Check sheet for the drawn part. Datum: minimum x, y, z corner. Units: mm. A direction names the side the tool comes from. Give positions to 0.01 mm unless a question says otherwise; leave off trailing zeros. Order: outer loops, then holes, each group sorted by start corner. A loop starts at its lowest first (then second) coordinate and runs counter-clockwise, first axis right, second up. Notation, with made-up numbers: M -0.5,-30.75 L 27.5,-30.75 A9 cw 27.5,-20.75 Z; hole C 12.25,72.5 d7. An arc over 180 degrees is marked long. Answer as CSV lines item,"result". Start each with the question number.
Q1. Section check A-A, the plane z = 24. Record the boundary of the cut face in (x, y), then the cut area to 3 significant figures.
Q2. Section check C-C, the plane x = 29. Record the boundary of the cut face in (y, z), then the cut area to 3 significant figures.
Q3. Thickness scan on line 1 (Z direction, x = 5, y = 8.25); line 2 (Y direction, x = 17, z = 19.5); line 3 (X direction, y = 17.5, z = 10.25). Record the ranges inside material, lowest first.
Q4. Set-up check for the marked faces 1, 2 and 3: record each of +Z, -Z, +X, -X, +Y, -Y from which the full face is reachable in a straight line by a thin tool's end or side.
Q5. Section check B-B, the plane x = 17. Record the boundary of the cut face in (y, z).
Q6. Go/stop test with flat-tipped pins: pin 1 (3.5 mm diameter, centred on y = 14.5, z = 20, fed in from -X); pin 2 (5.5 mm diameter, centred on x = 30.5, z = 21, fed in from +Y); pin 3 (5 mm diameter, centred on x = 8.5, z = 15.5, fed in from +Y). Record where each tip stops, or that it passes through.
Q7. Mould release check, pull along X, two halves, no side actions. Record for the marked faces 4, 5 and 6: +X half, -X half, draft (parallel to the pull), parting line (faces both ways), or undercut.
Q8. Section check D-D, the plane y = 13.25. Record the boundary of the cut face in (x, z), then the cut area to 3 significant figures.
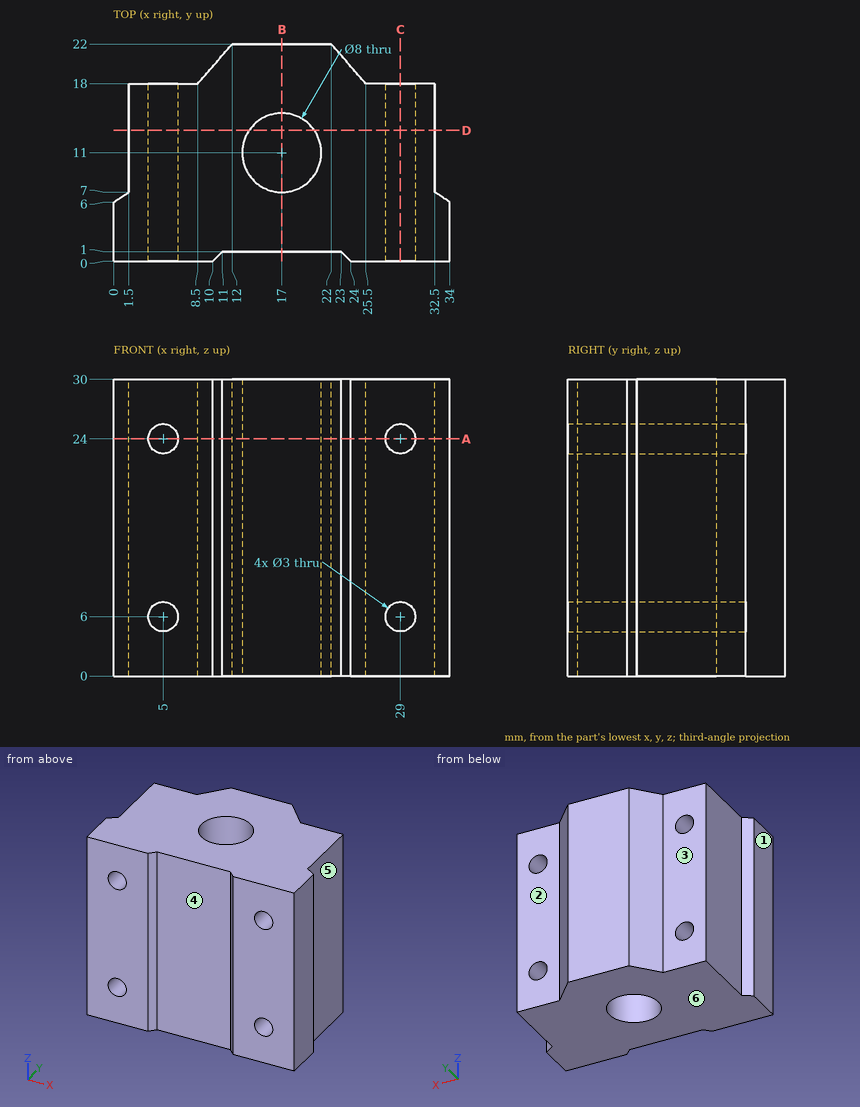
Answer block:
1,outline,"M 0,0 L 3.5,0 L 3.5,18 L 1.5,18 L 1.5,7 L 0,6 Z; M 6.5,0 L 10,0 L 11,1 L 23,1 L 24,0 L 27.5,0 L 27.5,18 L 25.5,18 L 22,22 L 12,22 L 8.5,18 L 6.5,18 Z; M 30.5,0 L 34,0 L 34,6 L 32.5,7 L 32.5,18 L 30.5,18 Z; hole C 17,11 d8"
1,area,"460 mm2"
2,outline,"M 0,0 L 18,0 L 18,4.5 L 0,4.5 Z; M 0,7.5 L 18,7.5 L 18,22.5 L 0,22.5 Z; M 0,25.5 L 18,25.5 L 18,30 L 0,30 Z"
2,area,"432 mm2"
3,line 1,"z = 0 to 4.5, 7.5 to 22.5, 25.5 to 30"
3,line 2,"y = 1 to 7, 15 to 22"
3,line 3,"x = 1.5 to 32.5"
4,face 1,"+Z, -Z, -X, +Y, -Y"
4,face 2,"+Z, -Z, +X, +Y"
4,face 3,"+Z, -Z, -X, +Y"
5,outline,"M 1,0 L 7,0 L 7,30 L 1,30 Z; M 15,0 L 22,0 L 22,30 L 15,30 Z"
6,pin 1,"stops at x = 1.5"
6,pin 2,"stops at y = 18"
6,pin 3,"stops at y = 20.86"
7,face 4,"undercut"
7,face 5,"+X half"
7,face 6,"draft"
8,outline,"M 1.5,0 L 13.69,0 L 13.69,30 L 1.5,30 Z; M 20.31,0 L 32.5,0 L 32.5,30 L 20.31,30 Z; hole C 5,6 d3; hole C 5,24 d3; hole C 29,6 d3; hole C 29,24 d3"
8,area,"703 mm2"
